from build123d import *

# Parameters (mm, degrees)
SKIZZE1_W                       = 179.5
SKIZZE1_H                       = 72
AUFSATZ_LINEAR_AUSTRAGEN1_DEPTH = 1.4
VERRUNDUNG1_R                   = 5
SKIZZE2_W                       = 24.97465075
SKIZZE2_H                       = 33
SCHNITT_LINEAR_AUSTRAGEN1_DEPTH = 97.711025742
SCHNITT_LINEAR_AUSTRAGEN2_DEPTH = 97.711025742
LINEARES_MUSTER1_COUNT          = 5
LINEARES_MUSTER1_PITCH          = 36


with BuildPart() as part:
    # Skizze1 → Aufsatz-Linear austragen1 (new body)
    with BuildSketch(Plane.XY):
        Rectangle(SKIZZE1_W, SKIZZE1_H)
    extrude(amount=AUFSATZ_LINEAR_AUSTRAGEN1_DEPTH)

    # Verrundung1
    verrundung1_edges = [part.edges().sort_by_distance(p)[0] for p in [
        (89.75, -36, 0.7),
        (-89.75, -36, 0.7),
        (-89.75, 36, 0.7),
        (89.75, 36, 0.7),
    ]]
    fillet(verrundung1_edges, radius=VERRUNDUNG1_R)

    # Skizze2 → Schnitt-Linear austragen1 (cut, through all)
    with BuildSketch(Plane.XY.offset(1.4)):
        with Locations((72, -14.487360935)):
            Rectangle(SKIZZE2_W, SKIZZE2_H)
    schnitt_linear_austragen1 = extrude(amount=-SCHNITT_LINEAR_AUSTRAGEN1_DEPTH, mode=Mode.SUBTRACT)

    # Skizze3 → Schnitt-Linear austragen2 (cut, through all)
    with BuildSketch(Plane.XY.offset(1.4)):
        Polygon((62.905000508, 28.468009652), (81.505000508, 28.468009652), (81.505000508, 27.968009652), (87.505000508, 27.968009652), (87.505000508, 4.818009652), (81.505000508, 4.818009652), (81.505000508, 4.168009652), (62.905000508, 4.168009652), (62.905000508, 4.818009652), (56.905000508, 4.818009652), (56.905000508, 27.968009652), (62.905000508, 27.968009652), align=None)
    schnitt_linear_austragen2 = extrude(amount=-SCHNITT_LINEAR_AUSTRAGEN2_DEPTH, mode=Mode.SUBTRACT)

    # Lineares Muster1: Schnitt-Linear austragen1, Schnitt-Linear austragen2 ×5
    with Locations(*[(-i * LINEARES_MUSTER1_PITCH, 0, 0) for i in range(1, LINEARES_MUSTER1_COUNT)]):
        add(schnitt_linear_austragen1, mode=Mode.SUBTRACT)
        add(schnitt_linear_austragen2, mode=Mode.SUBTRACT)


solid = part.part
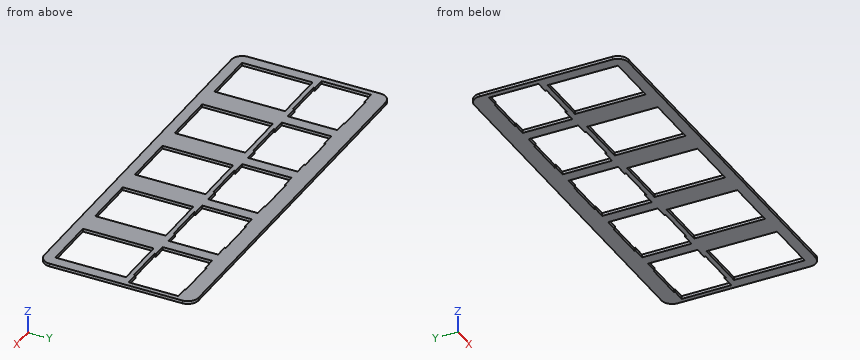
Geometry: final body of the model. Coordinates: model frame, mm. Round coordinates to 2 decimals unless told otherwise and drop trailing zeros. Order: outer loops, then holes, each group sorted by start corner. A loop starts at its lowest first (then second) coordinate and runs counter-clockwise, first axis right, second up. Notation, with made-up numbers: (-27.75, -21.75) -> (-11.75, -21.75) arc R18 ccw to (-11.75, -14.75) -> close; hole circle Ø5 at (60, 64.5). An arc over 180 degrees is marked (long way). Put each result on its own line as item: value. Start each with the question number.
Q1. Line query: probe 1 along X at (y, z) = (5, 0.2) (3 decimals); probe 2 along X at (y, z) = (-24.5, 1.35); probe 3 along Y at (x, z) = (60.5, 0.15). Output: solid intervals per line, ascending.
Q2. Section C-C on y = -0.5. Return the cut outline in (x, z).
Q3. Section B-B on x = -37.5. Return the cut outline in (y, z), and give its area (3 significant figures).
Q4. Section D-D on z = 0.35. Give the number of separate pieces and of enclosed holes in the cut face, and give its area (3 significant figures).
Q5. Section A-A on y = 16.5. Return the cut outline in (x, z) (3 decimals), and give its area (3 significant figures).
Ans:
1. probe 1: x = -89.75 to -87.095, -56.495 to -51.095, -20.495 to -15.095, 15.505 to 20.905, 51.505 to 56.905, 87.505 to 89.75
1. probe 2: x = -89.75 to -84.49, -59.51 to -48.49, -23.51 to -12.49, 12.49 to 23.51, 48.49 to 59.51, 84.49 to 89.75
1. probe 3: y = -36 to -30.99, 2.01 to 4.82, 27.97 to 36
2. outline: (-89.75, 0) -> (-84.49, 0) -> (-84.49, 1.4) -> (-89.75, 1.4) -> close; (-59.51, 0) -> (-48.49, 0) -> (-48.49, 1.4) -> (-59.51, 1.4) -> close; (-23.51, 0) -> (-12.49, 0) -> (-12.49, 1.4) -> (-23.51, 1.4) -> close; (12.49, 0) -> (23.51, 0) -> (23.51, 1.4) -> (12.49, 1.4) -> close; (48.49, 0) -> (59.51, 0) -> (59.51, 1.4) -> (48.49, 1.4) -> close; (84.49, 0) -> (89.75, 0) -> (89.75, 1.4) -> (84.49, 1.4) -> close
3. outline: (-36, 0) -> (-30.99, 0) -> (-30.99, 1.4) -> (-36, 1.4) -> close; (2.01, 0) -> (4.17, 0) -> (4.17, 1.4) -> (2.01, 1.4) -> close; (28.47, 0) -> (36, 0) -> (36, 1.4) -> (28.47, 1.4) -> close
3. area: 20.6 mm2
4. separate pieces: 1
4. enclosed holes: 10
4. area: 5,130 mm2
5. outline: (-89.75, 0) -> (-87.095, 0) -> (-87.095, 1.4) -> (-89.75, 1.4) -> close; (-56.495, 0) -> (-51.095, 0) -> (-51.095, 1.4) -> (-56.495, 1.4) -> close; (-20.495, 0) -> (-15.095, 0) -> (-15.095, 1.4) -> (-20.495, 1.4) -> close; (15.505, 0) -> (20.905, 0) -> (20.905, 1.4) -> (15.505, 1.4) -> close; (51.505, 0) -> (56.905, 0) -> (56.905, 1.4) -> (51.505, 1.4) -> close; (87.505, 0) -> (89.75, 0) -> (89.75, 1.4) -> (87.505, 1.4) -> close
5. area: 37.1 mm2
